The listing builds one solid part. Answer for the finished solid, in the listing's coordinates (mm). Round coordinates to 2 decimals unless told otherwise and drop trailing zeros. Write each loop counter-clockwise with the first axis right and the second up, starting at its lowest first coordinate (ties: lowest second). Pieces come first, ordered by that corner, then holes. Notation, with made-up numbers: (85, 1.25) - (112, 1.25) arc R17 ccw to (112, 12.25) - close; hole circle Ø5 at (87.5, 68.25). An arc over 180 degrees is marked (long way). Use a Markdown table: item, result. Add a question column.
1) A cutting plane is placed at B-B (z = 6). Give the vertices of the cut face in (x, y), then the cut area to 3 significant figures.
2) Determine the mould class of faces 1 (the cylindrical face through (6.38, 1.97, 7.71)), 2 (the flat face through (2, 2, 10)), 3 (the cylindrical face through (23.75, 1.97, 5.92)), 4 (the flat face through (14, 2, 0)) for opening direction Z: +Z half, -Z half, draft (parallel to the pull), parting line (faces both ways), or undercut.
3) Find the intervals of material crossed by probe 1 along X at (y, z) = (1.15, 6); probe 2 along Z at (x, y) = (22, 2.05); probe 3 along X at (y, z) = (1.9, 7), in increasing order. Write a range as from..to.
4) A cutting plane is placed at C-C (y = 1.7). Give the vertices of the cut face in (x, z).
5) A cutting plane is placed at D-D (z = 1). Give the vertices of the cut face in (x, y).
6) A cutting plane is placed at A-A (x = 22). Give the vertices of the cut face in (y, z).
```python
from build123d import *

# Parameters (mm, degrees)
BOSS_EXTRUDE1_DEPTH     = 12
SKETCH2_R               = 1.75
CUT_EXTRUDE1_DEPTH      = 1
CUT_EXTRUDE1_DEPTH_BACK = 5
CHAMFER1_SIZE           = 4


with BuildPart() as part:
    # Sketch1 → Boss-Extrude1 (new body)
    with BuildSketch(Plane.XY):
        Polygon((0, 0), (12, 0), (16, 0), (28, 0), (28, 4), (0, 4), align=None)
    extrude(amount=BOSS_EXTRUDE1_DEPTH)

    # Sketch2 → Cut-Extrude1 (cut, two sides)
    with BuildSketch(Plane(origin=(0, 0, 0), x_dir=(-1, 0, 0), z_dir=(0, -1, 0))) as cut_extrude1_sk:
        with Locations((-6, -6)):
            Circle(SKETCH2_R)
        with Locations((-22, -6)):
            Circle(SKETCH2_R)
    extrude(amount=CUT_EXTRUDE1_DEPTH, mode=Mode.SUBTRACT)
    extrude(cut_extrude1_sk.sketch, amount=-CUT_EXTRUDE1_DEPTH_BACK, mode=Mode.SUBTRACT)

    # Chamfer1
    chamfer1_edges = [part.edges().sort_by_distance(p)[0] for p in [
        (28, 2, 12),
        (0, 2, 12),
        (28, 2, 0),
        (0, 2, 0),
    ]]
    chamfer(chamfer1_edges, length=CHAMFER1_SIZE)


solid = part.part
```
Entries:
| question | item | result |
|---|---|---|
| 1 | outline | (0, 0) - (4.25, 0) - (4.25, 4) - (0, 4) - close; (7.75, 0) - (20.25, 0) - (20.25, 4) - (7.75, 4) - close; (23.75, 0) - (28, 0) - (28, 4) - (23.75, 4) - close |
| 1 | area | 84.0 mm² |
| 2 | face 1 | undercut |
| 2 | face 2 | +Z half |
| 2 | face 3 | undercut |
| 2 | face 4 | -Z half |
| 3 | probe 1 | x = 0..4.25, 7.75..20.25, 23.75..28 |
| 3 | probe 2 | z = 0..4.25, 7.75..12 |
| 3 | probe 3 | x = 0..4.56, 7.44..20.56, 23.44..28 |
| 4 | outline | (0, 4) - (4, 0) - (24, 0) - (28, 4) - (28, 8) - (24, 12) - (4, 12) - (0, 8) - close; hole circle Ø3.5 at (6, 6); hole circle Ø3.5 at (22, 6) |
| 5 | outline | (3, 0) - (25, 0) - (25, 4) - (3, 4) - close |
| 6 | outline | (0, 0) - (4, 0) - (4, 4.25) - (0, 4.25) - close; (0, 7.75) - (4, 7.75) - (4, 12) - (0, 12) - close |
